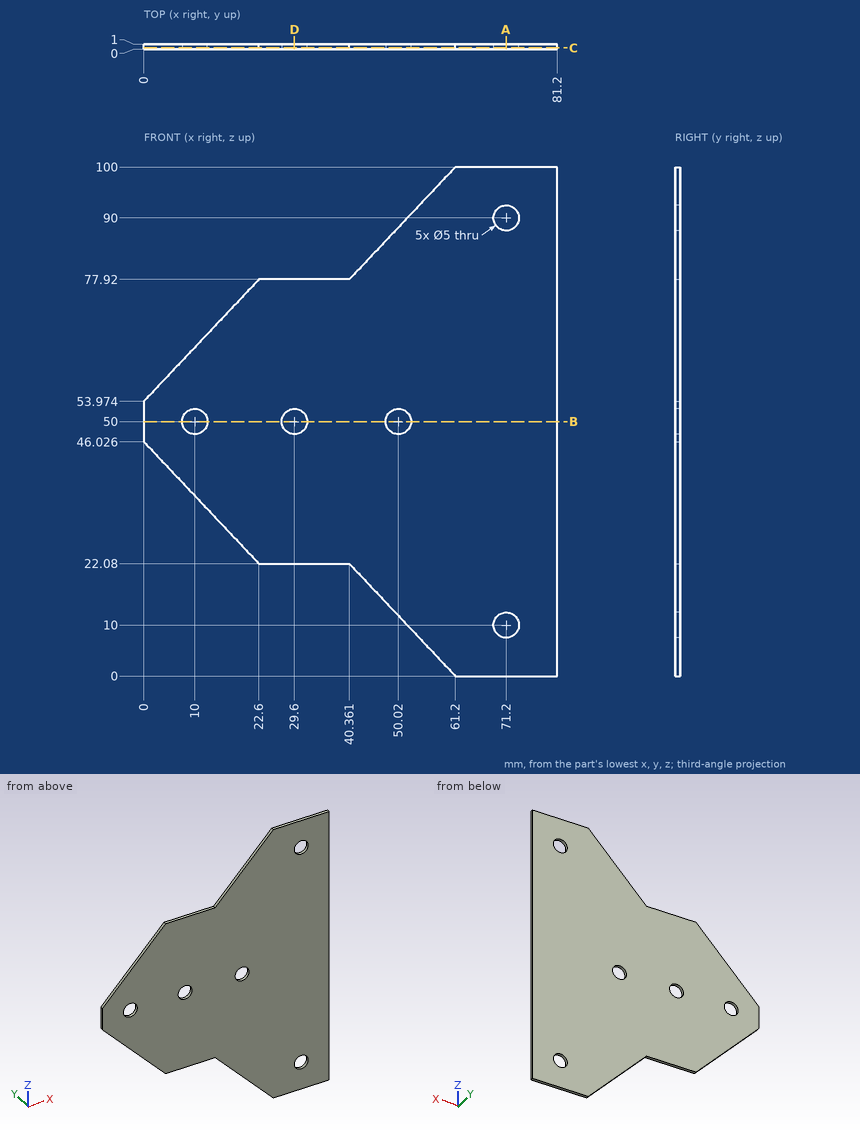
Job drawing, mm, ordinate dimensions from the low corner. One solid piece. Coordinates: 2 decimals unless noted, no trailing zeros. Order: outer loops, then holes, each group sorted by start corner. A loop starts at its lowest first (then second) coordinate and runs counter-clockwise, first axis right, second up. Notation, with made-up numbers: M 45,2.5 L 54,2.5 A6 ccw 54,9.5 Z; hole C 33.25,70.5 d9. An arc over 180 degrees is marked long. Answer as CSV lines item,"result".
(1) Band-saw the part on C-C, the plane y = 0.25. List the corners of the cut face in (x, z), then the cut area to 3 significant figures.
Geometry says:
outline,"M 0,46.03 L 22.6,22.08 L 40.36,22.08 L 61.2,0 L 81.2,0 L 81.2,100 L 61.2,100 L 40.36,77.92 L 22.6,77.92 L 0,53.97 Z; hole C 10,50 d5; hole C 29.6,50 d5; hole C 50.02,50 d5; hole C 71.2,10 d5; hole C 71.2,90 d5"
area,"5,240 mm2"
(2) Wall check: line 1 along X through (y, z) = (0.65, 50); line 2 along Z through (x, y) = (71.2, 0.8); line 3 along Z through (x, y) = (29.6, 0.75). Give the ranges that are in metal, low to high.
Geometry says:
line 1,"x = 0 to 7.5, 12.5 to 27.1, 32.1 to 47.52, 52.52 to 81.2"
line 2,"z = 0 to 7.5, 12.5 to 87.5, 92.5 to 100"
line 3,"z = 22.08 to 47.5, 52.5 to 77.92"
(3) Band-saw the part on A-A, the plane x = 71.2. List the corners of the cut face in (y, z).
Geometry says:
outline,"M 0,0 L 1,0 L 1,7.5 L 0,7.5 Z; M 0,12.5 L 1,12.5 L 1,87.5 L 0,87.5 Z; M 0,92.5 L 1,92.5 L 1,100 L 0,100 Z"
(4) Band-saw the part on B-B, the plane z = 50. List the corners of the cut face in (x, y).
Geometry says:
outline,"M 0,0 L 7.5,0 L 7.5,1 L 0,1 Z; M 12.5,0 L 27.1,0 L 27.1,1 L 12.5,1 Z; M 32.1,0 L 47.52,0 L 47.52,1 L 32.1,1 Z; M 52.52,0 L 81.2,0 L 81.2,1 L 52.52,1 Z"
(5) Band-saw the part on D-D, the plane x = 29.6. List the corners of the cut face in (y, z).
Geometry says:
outline,"M 0,22.08 L 1,22.08 L 1,47.5 L 0,47.5 Z; M 0,52.5 L 1,52.5 L 1,77.92 L 0,77.92 Z"
(6) Flat gauge pins, fed straight in: pin 1 (1 mm diameter, centred on x = 32, z = 55, fed in from -Y); pin 2 (0.5 mm diameter, centred on x = 32, y = 0.5, fed in from +Z). Where does each tip first touch, or does it go through?
Geometry says:
pin 1,"stops at y = 0"
pin 2,"stops at z = 77.92"
